The model under review builds one solid part; all positions refer to its coordinate system, in mm. Face numbers are marked on the shaded views. Coordinates: 2 decimals unless noted, no trailing zeros. Write each loop counter-clockwise with the first axis right and the second up, starting at its lowest first coordinate (ties: lowest second). Pieces come first, ordered by that corner, then holes. Notation, with made-up numbers: M 18.25,54 L 25.25,54 A18 ccw 25.25,63 Z; hole C 69,60.5 d9. An arc over 180 degrees is marked long. Answer as a JSON object with one key per item and string values.
```python
from build123d import *

# Parameters (mm, degrees)
EXTRUDE_START        = 10
SKETCH_1_R           = 2.5
EXTRUDE_1_DEPTH      = 5
EXTRUDE_2_DEPTH      = 6
EXTRUDE_2_DEPTH_BACK = 6
SKETCH_2_R           = 2.25


with BuildPart() as part:
    # Эскиз1 → Бобышка-Вытянуть1 (new body)
    with BuildSketch(Plane.XY.offset(EXTRUDE_START)):
        Circle(SKETCH_1_R)
    extrude_1 = extrude(amount=-EXTRUDE_1_DEPTH)

    # Эскиз2 → Бобышка-Вытянуть2 (add, two sides: drawn at the far end of the back side and taken through both)
    with BuildSketch(Plane.XY.offset(-EXTRUDE_2_DEPTH_BACK)):
        Circle(SKETCH_2_R)
    extrude(amount=EXTRUDE_2_DEPTH + EXTRUDE_2_DEPTH_BACK)

    # Зеркальное отражение1: Бобышка-Вытянуть1 across plane
    add(extrude_1.mirror(Plane.XY))


solid = part.part
```
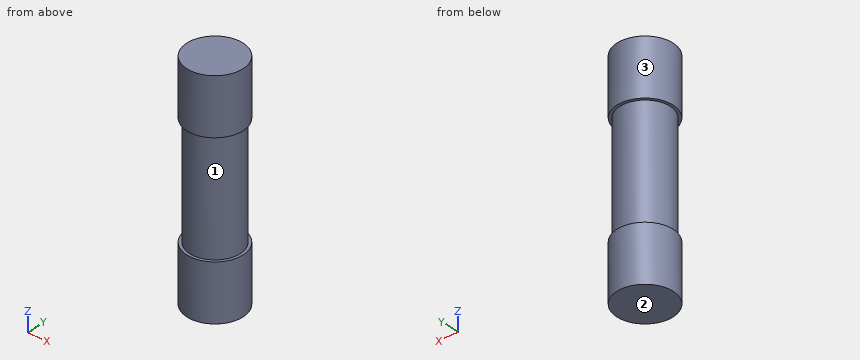
(1) Draft analysis for pull direction Z (two halves, no side actions). For the marked faces 1, 2 and 3, state which applies: released by +Z, released by -Z, zero draft, split by the parting line, or undercut.
Results list:
{"face 1": "undercut", "face 2": "released by -Z", "face 3": "zero draft"}
(2) Wall thickness on line 1 along Z through (x, y) = (1.8, -1.7); line 2 along X through (y, z) = (-0.1, 0); line 3 along X through (y, z) = (1.7, 2.75): over which ranges is each line inside the solid? List them lowest first. Write a range as from..to.
Results list:
{"line 1": "-10..-5, 5..10", "line 2": "-2.25..2.25", "line 3": "-1.47..1.47"}
(3) Add section A-A on y = 0. Give the boundary of the cut face in (x, z), and give its area (3 significant figures).
Results list:
{"outline": "M -2.5,-10 L 2.5,-10 L 2.5,-5 L 2.25,-5 L 2.25,5 L 2.5,5 L 2.5,10 L -2.5,10 L -2.5,5 L -2.25,5 L -2.25,-5 L -2.5,-5 Z", "area": "95.0 mm²"}
(4) Add section D-D on z = 8.25. Give the boundary of the cut face in (x, y), and give its area (3 significant figures).
Results list:
{"outline": "C 0,0 d5", "area": "19.6 mm²"}
(5) Add section B-B on x = 0.95. Give the boundary of the cut face in (y, z), and give its area (3 significant figures).
Results list:
{"outline": "M -2.31,-10 L 2.31,-10 L 2.31,-5 L 2.04,-5 L 2.04,5 L 2.31,5 L 2.31,10 L -2.31,10 L -2.31,5 L -2.04,5 L -2.04,-5 L -2.31,-5 Z", "area": "87.0 mm²"}
(6) Add section C-C on z = 4. Give the boundary of the cut face in (x, y).
Results list:
{"outline": "C 0,0 d4.5"}
